The model under review builds one solid part; all positions refer to its coordinate system, in mm. A direction names the side the tool comes from. Coordinates: 2 decimals unless noted, no trailing zeros. Loops run counter-clockwise (first coordinate to the right, second up) from the corner with the lowest first, then second, coordinate; pieces in that order, holes last. Notation, with made-up numbers: M 36,-22.5 L 44,-22.5 A28 cw 44,-3.5 Z; hole C 55.25,44 d5. An arc over 180 degrees is marked long. Return JSON: item names as keys, results as strings.
```python
from build123d import *

# Parameters (mm, degrees)
SALIENTE_EXTRUIR1_DEPTH = 90
CROQUIS2_W              = 90
CROQUIS2_H              = 350
SALIENTE_EXTRUIR2_DEPTH = 12.7


with BuildPart() as part:
    # Croquis1 → Saliente-Extruir1 (new body)
    with BuildSketch(Plane.XY):
        with BuildLine():
            Line((0, 0), (0, 100))
            Line((0, 100), (10, 100))
            Line((10, 100), (10, 14))
            ThreePointArc((10, 14), (11.171572875, 11.171572875), (14, 10))
            Line((14, 10), (100, 10))
            Line((100, 10), (100, 0))
            Line((100, 0), (0, 0))
        make_face()
    extrude(amount=SALIENTE_EXTRUIR1_DEPTH)

    # Croquis2 → Saliente-Extruir2 (add)
    with BuildSketch(Plane.ZY):
        with Locations((45, 175)):
            Rectangle(CROQUIS2_W, CROQUIS2_H)
    extrude(amount=SALIENTE_EXTRUIR2_DEPTH)


solid = part.part
```
1. Add section C-C on x = 46. Give the boundary of the cut face in (y, z).
Check values:
{"outline": "M 0,0 L 10,0 L 10,90 L 0,90 Z"}
2. Add section A-A on z = 11.5. Give the boundary of the cut face in (x, y).
Check values:
{"outline": "M -12.7,0 L 100,0 L 100,10 L 14,10 A4 cw 10,14 L 10,100 L 0,100 L 0,350 L -12.7,350 Z"}
3. Add section B-B on y = 86. Give the boundary of the cut face in (x, z), plus the area to 3 significant figures.
Check values:
{"outline": "M -12.7,0 L 10,0 L 10,90 L -12.7,90 Z", "area": "2,040 mm²"}
4. The part is to be moulded in two halves that separate along X. For faces 1 (the face through (0, 227, 44)), 2 (the face through (44, 0, 44)), 3 (the face through (-12.7, 177, 44)), say which applies: released by +X, released by -X, zero draft, split by the parting line, or undercut.
Check values:
{"face 1": "released by +X", "face 2": "zero draft", "face 3": "released by -X"}
5. Machinability: for faces 4 (the face through (-2, 122, 0)), 5 (the face through (10, 58, 44)), which of the approach directions +Z, -Z, +X, -X, +Y, -Y give a long, thin tool a straight path to every point of the face, cutting with its end or side? Answer none if there is none.
Check values:
{"face 4": "-Z, +X, -X, +Y, -Y", "face 5": "+Z, -Z, +X, +Y"}
6. Insertion check: pin 1 Ø4 at (y, z) = (156.5, 18) entering from +X; pin 2 Ø12 at (x, z) = (65, 78) entering from +Y. Each pin has a flat end and moves straight along its axis. Give the tip position at first contact, or say it passes through.
Check values:
{"pin 1": "x = 0", "pin 2": "y = 10"}
7. To check wall thickness, follow line 1 (Y direction, x = 82, z = 84.5); line 2 (X direction, y = 213.5, z = 36); line 3 (Y direction, x = 4.5, z = 53). State the ranges of each line that lie inside material, in increasing order.
Check values:
{"line 1": "0 to 10", "line 2": "-12.7 to 0", "line 3": "0 to 100"}
